Could you check a few things on this model? Use its own coordinates, in mm. Face numbers are marked on the shaded views. A direction names the side the tool comes from. Give positions to 0.01 mm unless a question says otherwise; leave off trailing zeros. Order: outer loops, then holes, each group sorted by start corner. A loop starts at its lowest first (then second) coordinate and runs counter-clockwise, first axis right, second up. Notation, with made-up numbers: M 49,9 L 98,9 A3 ccw 98,13 Z; hole C 49,59.25 d5. An arc over 180 degrees is marked long. Use a Markdown table: item, result. Add a question column.
Item 1: If we mould it in two halves opening along Y, with no side actions, what happens to the marked faces 3, 4 and 5? For each: released by +Y, released by -Y, zero draft, split by the parting line, or undercut.
Item 2: Suppose I cut it at A-A on y = -19.05. Write out the boundary of the cut face in (x, z), plus the area to 3 significant figures.
Item 3: For the marked faces 1 and 2, which set-ups out of +Z, -Z, +X, -X, +Y, -Y let a thin tool reach every point of the face, with its end or its side?
Item 4: I'm going to push flat-ended pins straight in: pin 1 Ø12.5 at (y, z) = (-39, -40.5) entering from +X; pin 2 Ø9.5 at (y, z) = (-65.89, -69.06) entering from -X; pin 3 Ø23 at (y, z) = (-34.92, -38.11) entering from -X; pin 4 Ø1.1 at (y, z) = (-17.23, -20.41) entering from +X. Where does each tip first touch, or does it pass through?
Item 5: Suppose I cut it at B-B on y = -65. Write out the boundary of the cut face in (x, z).
Item 6: Suppose I cut it at C-C on z = -29.5. Count the separate pieces of the cut face and the enclosed holes in it, plus the area to 3 significant figures.
Item 7: If I drill on L1, parallel to Y at x = 6.5, z = -58.5 (3 decimals); L2, parallel to Y at x = 5, z = -40 (3 decimals); L3, parallel to Z at x = 12, y = -66, over which ranges is the centre line in solid material (lowest first)? Write a range as from..to.
from build123d import *

# Parameters (mm, degrees)
SKETCH1_W          = 76.2
SKETCH1_H          = 73.025
EXTRUDE1_DEPTH     = 12.7
SKETCH8_R          = 0.889
SKETCH8_R_2        = 3.175
SKETCH8_R_3        = 7.112
SKETCH8_R_4        = 2.38125
CUT_EXTRUDE5_DEPTH = 12.7
SKETCH11_R         = 5.207
CUT_EXTRUDE6_DEPTH = 6.35
SKETCH13_R         = 17.4625
CUT_EXTRUDE7_DEPTH = 4.2545
SKETCH14_R         = 12.7
CUT_EXTRUDE8_DEPTH = 0.254
SKETCH15_R         = 2.0193
CUT_EXTRUDE9_DEPTH = 77.2


with BuildPart() as part:
    # Sketch1 → Extrude1 (new body)
    with BuildSketch(Plane(origin=(0, 0, 0), x_dir=(0, 0, -1), z_dir=(1, 0, 0))):
        with Locations((38.1, -36.5125)):
            Rectangle(SKETCH1_W, SKETCH1_H)
    extrude(amount=EXTRUDE1_DEPTH)

    # Sketch8 → Cut-Extrude5 (cut)
    with BuildSketch(Plane.ZY):
        with Locations((-55.796122625, -17.233895441)):
            Circle(SKETCH8_R)
        with Locations((-7.1374, -7.1374)):
            Circle(SKETCH8_R_2)
        with Locations((-69.0626, -7.1374)):
            Circle(SKETCH8_R_2)
        with Locations((-69.0626, -65.8876)):
            Circle(SKETCH8_R_2)
        with Locations((-7.1374, -65.8876)):
            Circle(SKETCH8_R_2)
        with Locations((-38.105018066, -34.925)):
            Circle(SKETCH8_R_3)
        with Locations((-69.0626, -34.925)):
            Circle(SKETCH8_R_4)
        with Locations((-7.1374, -34.925)):
            Circle(SKETCH8_R_4)
        with Locations((-20.413913508, -17.233895441)):
            Circle(SKETCH8_R)
        with Locations((-55.796122625, -52.616104559)):
            Circle(SKETCH8_R)
        with Locations((-20.413913508, -52.616104559)):
            Circle(SKETCH8_R)
    extrude(amount=-CUT_EXTRUDE5_DEPTH, mode=Mode.SUBTRACT)

    # Sketch11 → Cut-Extrude6 (cut)
    with BuildSketch(Plane.ZY):
        with Locations((-7.1374, -7.1374)):
            Circle(SKETCH11_R)
        with Locations((-69.0626, -7.1374)):
            Circle(SKETCH11_R)
        with Locations((-69.0626, -65.8876)):
            Circle(SKETCH11_R)
        with Locations((-7.1374, -65.8876)):
            Circle(SKETCH11_R)
    extrude(amount=-CUT_EXTRUDE6_DEPTH, mode=Mode.SUBTRACT)

    # Sketch13 → Cut-Extrude7 (cut)
    with BuildSketch(Plane.ZY):
        with Locations((-38.105018066, -34.925)):
            Circle(SKETCH13_R)
    extrude(amount=-CUT_EXTRUDE7_DEPTH, mode=Mode.SUBTRACT)

    # Sketch14 → Cut-Extrude8 (cut)
    with BuildSketch(Plane(origin=(12.7, 0, 0), x_dir=(0, 0, -1), z_dir=(1, 0, 0))):
        with Locations((38.105018066, -34.925)):
            Circle(SKETCH14_R)
    extrude(amount=-CUT_EXTRUDE8_DEPTH, mode=Mode.SUBTRACT)

    # Sketch15 → Cut-Extrude9 (cut, through all)
    with BuildSketch(Plane(origin=(0, 0, 0), x_dir=(-1, 0, 0), z_dir=(0, 0, -1))):
        with Locations((-6.35, -19.05)):
            Circle(SKETCH15_R)
        with Locations((-6.35, -53.975)):
            Circle(SKETCH15_R)
    extrude(amount=CUT_EXTRUDE9_DEPTH, mode=Mode.SUBTRACT)


solid = part.part
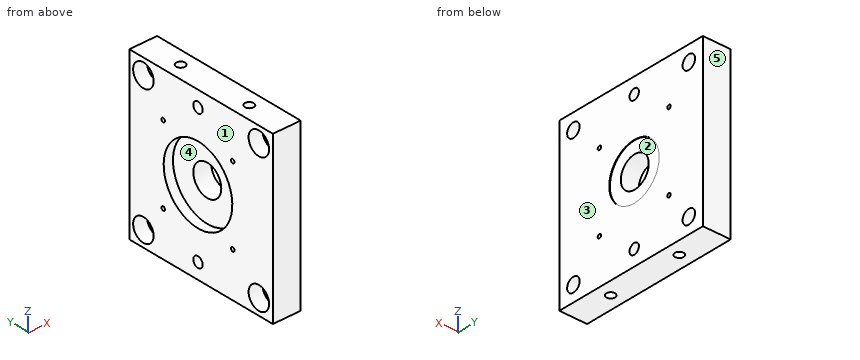
Findings below:
| question | item | result |
|---|---|---|
| 1 | face 3 | zero draft |
| 1 | face 4 | undercut |
| 1 | face 5 | released by +Y |
| 2 | outline | M 0,-76.2 L 4.33,-76.2 L 4.33,0 L 0,0 L 0,-30.83 L 4.25,-30.83 L 4.25,-45.38 L 0,-45.38 Z; M 8.37,-76.2 L 12.7,-76.2 L 12.7,0 L 8.37,0 Z |
| 2 | area | 598 mm^2 |
| 3 | face 1 | +Z, -Z, -X, +Y, -Y |
| 3 | face 2 | +X |
| 4 | pin 1 | stops at x = 12.45 |
| 4 | pin 2 | stops at x = 6.35 |
| 4 | pin 3 | stops at x = 4.25 |
| 4 | pin 4 | passes through |
| 5 | outline | M 0,-76.2 L 12.7,-76.2 L 12.7,-72.11 L 6.35,-72.11 L 6.35,-74.19 L 0,-74.19 Z; M 0,-63.93 L 6.35,-63.93 L 6.35,-66.01 L 12.7,-66.01 L 12.7,-10.19 L 6.35,-10.19 L 6.35,-12.27 L 0,-12.27 Z; M 0,-2.01 L 6.35,-2.01 L 6.35,-4.09 L 12.7,-4.09 L 12.7,0 L 0,0 Z |
| 6 | separate pieces | 1 |
| 6 | enclosed holes | 2 |
| 6 | area | 768 mm^2 |
| 7 | L1 | y = -73.025..-55.989, -51.961..-21.064, -17.036..0 |
| 7 | L2 | y = -73.025..-55.477, -52.473..-41.78, -28.07..-20.552, -17.548..0 |
| 7 | L3 | z = -76.2..-72.24, -65.89..-10.31, -3.96..0 |
